```python
from build123d import *

# Parameters (mm, degrees)
F0_R     = 50.8
F1_DEPTH = 25.4
F2_W     = 19.05
F2_H     = 95.25
F3_DEPTH = 12.7
F5_DEPTH = 25.4


with BuildPart() as f1:
    # F0 (on Top) → F1 (new body)
    with BuildSketch(Plane.XY):
        Circle(F0_R)
    extrude(amount=F1_DEPTH)

    # F2 (on face) → F3 (cut)
    with BuildSketch(Plane(origin=(0, 0, 0), x_dir=(1, 0, 0), z_dir=(0, 0, -1))):
        Rectangle(F2_W, F2_H)
    extrude(amount=-F3_DEPTH, mode=Mode.SUBTRACT)

    # F4 (on face) → F5 (cut)
    with BuildSketch(Plane.XY.offset(25.4)):
        with BuildLine():
            Line((3.387666, 3.347405), (-3.387666, 3.347405))
            ThreePointArc((-3.387666, 3.347405), (0, -4.7625), (3.387666, 3.347405))
        make_face()
    extrude(amount=-F5_DEPTH, mode=Mode.SUBTRACT)


solid = f1.part
```
Design review of the part built by this model. Coordinates are the model's own, in mm. A direction names the side the tool comes from. Coordinates: 2 decimals unless noted, no trailing zeros. Loops run counter-clockwise (first coordinate to the right, second up) from the corner with the lowest first, then second, coordinate; pieces in that order, holes last. Notation, with made-up numbers: M 61,-0.75 L 92,-0.75 A30 cw 92,29.25 Z; hole C -21,-25.75 d6. An arc over 180 degrees is marked long. One line per question, with ' | ' between items.
(1) Machinability: for faces 5 (the face through (-0.16, -4.76, 19.14)), 6 (the face through (0, 47.625, 6)), which of the approach directions +Z, -Z, +X, -X, +Y, -Y give a long, thin tool a straight path to every point of the face, cutting with its end or side? Answer none if there is none.
Filled in:
face 5: +Z, -Z | face 6: -Z
(2) We need section B-B (y = 0). Give the boundary of the cut face in (x, z) (1 decimal), and give its area (3 significant figures).
Filled in:
outline: M -50.8,0 L -9.5,0 L -9.5,12.7 L -4.8,12.7 L -4.8,25.4 L -50.8,25.4 Z; M 4.8,12.7 L 9.5,12.7 L 9.5,0 L 50.8,0 L 50.8,25.4 L 4.8,25.4 Z | area: 2,220 mm^2
(3) We need section D-D (y = -43). Give the boundary of the cut face in (x, z) (3 decimals).
Filled in:
outline: M -27.049,0 L -9.525,0 L -9.525,12.7 L 9.525,12.7 L 9.525,0 L 27.049,0 L 27.049,25.4 L -27.049,25.4 Z
(4) We need section C-C (z = 6.5). Give the boundary of the cut face in (x, y) (3 decimals), and give its area (3 significant figures).
Filled in:
outline: C 0,0 d101.6; hole M -9.525,-47.625 L 9.525,-47.625 L 9.525,47.625 L -9.525,47.625 Z | area: 6,290 mm^2
(5) For pin 1 Ø4 at (y, z) = (16.5, 5.5) entering from -X; pin 2 Ø8 at (x, z) = (13.5, 17) entering from +Y; pin 3 Ø1 at (y, z) = (19, 16.5) entering from +X, all flat-tipped, find the tip position at first contact; note any pin that passes through.
Filled in:
pin 1: stops at x = -48.69 | pin 2: stops at y = 49.9 | pin 3: stops at x = 47.31
(6) Wall thickness on probe 1 along X at (y, z) = (1, 1.75) (3 decimals); probe 2 along Y at (x, z) = (0, 20); probe 3 along X at (y, z) = (-39.5, 4) (3 decimals): over which ranges is each line inside the solid? List them lowest first.
Filled in:
probe 1: x = -50.79 to -9.525, 9.525 to 50.79 | probe 2: y = -50.8 to -4.76, 3.35 to 50.8 | probe 3: x = -31.944 to -9.525, 9.525 to 31.944
(7) Draft analysis for pull direction X (two halves, no side actions). For faces 1 (the face through (9.525, 1, 6)), 2 (the face through (11, 1, 0)), 3 (the face through (0, 3.347, 19)), 4 (the face through (-11.012, -49.592, 12.522)), state which applies: released by +X, released by -X, zero draft, split by the parting line, or undercut.
Filled in:
face 1: undercut | face 2: zero draft | face 3: undercut | face 4: split by the parting line
(8) We need section A-A (x = 0). Give the boundary of the cut face in (y, z) (1 decimal), and give its area (3 significant figures).
Filled in:
outline: M -50.8,0 L -47.6,0 L -47.6,12.7 L -4.8,12.7 L -4.8,25.4 L -50.8,25.4 Z; M 3.3,12.7 L 47.6,12.7 L 47.6,0 L 50.8,0 L 50.8,25.4 L 3.3,25.4 Z | area: 1,270 mm^2
